```python
from build123d import *

# Parameters (mm, degrees)
F0_W      = 25.4
F0_H      = 25.580178
F2_DEPTH  = 25.4
F1_R      = 1.8161
F3_DEPTH  = 11.2776
F1_R_2    = 11.5316
F1_R_3    = 8.382
F4_DEPTH  = 3.7338
F1_R_4    = 4.9911
F5_DEPTH  = 8.8138
F6_DEPTH  = 6.1722
F7_R      = 1.8161
F12_DEPTH = 11.2776
F8_R      = 1.8161
F13_DEPTH = 11.2776
F9_R      = 1.8161
F14_DEPTH = 11.2776
F11_R     = 1.8161
F15_DEPTH = 11.2776
F10_R     = 1.8161
F16_DEPTH = 11.2776
F9_R_2    = 4.9911
F17_DEPTH = 8.8138
F11_R_2   = 4.9911
F18_DEPTH = 8.8138
F11_R_3   = 8.382
F19_DEPTH = 6.1722
F11_R_4   = 11.5316
F20_DEPTH = 3.7338
F21_DEPTH = 8.8138
F9_R_3    = 8.382
F22_DEPTH = 6.1722
F9_R_4    = 11.5316
F23_DEPTH = 3.7338
F10_R_2   = 4.9911
F24_DEPTH = 8.8138
F10_R_3   = 8.382
F25_DEPTH = 6.1722
F10_R_4   = 11.5316
F26_DEPTH = 3.7338
F8_R_2    = 4.9911
F27_DEPTH = 8.8138
F8_R_3    = 8.382
F28_DEPTH = 6.1722
F7_R_2    = 4.9911
F29_DEPTH = 8.8138
F7_R_3    = 8.382
F30_DEPTH = 6.1722
F7_R_4    = 11.5316
F31_DEPTH = 3.7338
F8_R_4    = 11.5316
F32_DEPTH = 3.7338


with BuildPart() as f2:
    # F0 (on Front) → F2 (new body)
    with BuildSketch(Plane.XZ):
        Rectangle(F0_W, F0_H)
    extrude(amount=-F2_DEPTH)

    # F1 (on Front) → F3 (cut)
    with BuildSketch(Plane.XZ):
        Circle(F1_R)
    extrude(amount=-F3_DEPTH, mode=Mode.SUBTRACT)

    # F1 (on Front) → F4 (cut)
    with BuildSketch(Plane.XZ):
        Circle(F1_R_2)
        Circle(F1_R_3, mode=Mode.SUBTRACT)
    extrude(amount=-F4_DEPTH, mode=Mode.SUBTRACT)

    # F1 (on Front) → F5 (cut)
    with BuildSketch(Plane.XZ):
        Circle(F1_R_4)
        Circle(F1_R, mode=Mode.SUBTRACT)
    extrude(amount=-F5_DEPTH, mode=Mode.SUBTRACT)

    # F1 (on Front) → F6 (cut)
    with BuildSketch(Plane.XZ):
        Circle(F1_R_3)
        Circle(F1_R_4, mode=Mode.SUBTRACT)
    extrude(amount=-F6_DEPTH, mode=Mode.SUBTRACT)

    # F7 (on face) → F12 (cut)
    with BuildSketch(Plane(origin=(-12.7, 0, 0), x_dir=(0, -1, 0), z_dir=(-1, 0, 0))):
        with Locations((-12.7, 0)):
            Circle(F7_R)
    extrude(amount=-F12_DEPTH, mode=Mode.SUBTRACT)

    # F8 (on face) → F13 (cut)
    with BuildSketch(Plane(origin=(0, 0, -12.790089), x_dir=(1, 0, 0), z_dir=(0, 0, -1))):
        with Locations((0, -12.7)):
            Circle(F8_R)
    extrude(amount=-F13_DEPTH, mode=Mode.SUBTRACT)

    # F9 (on face) → F14 (cut)
    with BuildSketch(Plane.XY.offset(12.790089)):
        with Locations((0, 12.7)):
            Circle(F9_R)
    extrude(amount=-F14_DEPTH, mode=Mode.SUBTRACT)

    # F11 (on face) → F15 (cut)
    with BuildSketch(Plane(origin=(0, 25.4, 0), x_dir=(-1, 0, 0), z_dir=(0, 1, 0))):
        Circle(F11_R)
    extrude(amount=-F15_DEPTH, mode=Mode.SUBTRACT)

    # F10 (on face) → F16 (cut)
    with BuildSketch(Plane.YZ.offset(12.7)):
        with Locations((12.7, 0)):
            Circle(F10_R)
    extrude(amount=-F16_DEPTH, mode=Mode.SUBTRACT)

    # F9 (on face) → F17 (cut)
    with BuildSketch(Plane.XY.offset(12.790089)):
        with Locations((0, 12.7)):
            Circle(F9_R_2)
        with Locations((0, 12.7)):
            Circle(F9_R, mode=Mode.SUBTRACT)
    extrude(amount=-F17_DEPTH, mode=Mode.SUBTRACT)

    # F11 (on face) → F18 (cut)
    with BuildSketch(Plane(origin=(0, 25.4, 0), x_dir=(-1, 0, 0), z_dir=(0, 1, 0))):
        Circle(F11_R_2)
        Circle(F11_R, mode=Mode.SUBTRACT)
    extrude(amount=-F18_DEPTH, mode=Mode.SUBTRACT)

    # F11 (on face) → F19 (cut)
    with BuildSketch(Plane(origin=(0, 25.4, 0), x_dir=(-1, 0, 0), z_dir=(0, 1, 0))):
        Circle(F11_R_3)
        Circle(F11_R_2, mode=Mode.SUBTRACT)
    extrude(amount=-F19_DEPTH, mode=Mode.SUBTRACT)

    # F11 (on face) → F20 (cut)
    with BuildSketch(Plane(origin=(0, 25.4, 0), x_dir=(-1, 0, 0), z_dir=(0, 1, 0))):
        Circle(F11_R_4)
        Circle(F11_R_3, mode=Mode.SUBTRACT)
    extrude(amount=-F20_DEPTH, mode=Mode.SUBTRACT)

    # F9 (on face) → F21 (cut)
    with BuildSketch(Plane.XY.offset(12.790089)):
        with Locations((0, 12.7)):
            Circle(F9_R_2)
        with Locations((0, 12.7)):
            Circle(F9_R, mode=Mode.SUBTRACT)
    extrude(amount=-F21_DEPTH, mode=Mode.SUBTRACT)

    # F9 (on face) → F22 (cut)
    with BuildSketch(Plane.XY.offset(12.790089)):
        with Locations((0, 12.7)):
            Circle(F9_R_3)
        with Locations((0, 12.7)):
            Circle(F9_R_2, mode=Mode.SUBTRACT)
    extrude(amount=-F22_DEPTH, mode=Mode.SUBTRACT)

    # F9 (on face) → F23 (cut)
    with BuildSketch(Plane.XY.offset(12.790089)):
        with Locations((0, 12.7)):
            Circle(F9_R_4)
        with Locations((0, 12.7)):
            Circle(F9_R_3, mode=Mode.SUBTRACT)
    extrude(amount=-F23_DEPTH, mode=Mode.SUBTRACT)

    # F10 (on face) → F24 (cut)
    with BuildSketch(Plane.YZ.offset(12.7)):
        with Locations((12.7, 0)):
            Circle(F10_R_2)
        with Locations((12.7, 0)):
            Circle(F10_R, mode=Mode.SUBTRACT)
    extrude(amount=-F24_DEPTH, mode=Mode.SUBTRACT)

    # F10 (on face) → F25 (cut)
    with BuildSketch(Plane.YZ.offset(12.7)):
        with Locations((12.7, 0)):
            Circle(F10_R_3)
        with Locations((12.7, 0)):
            Circle(F10_R_2, mode=Mode.SUBTRACT)
    extrude(amount=-F25_DEPTH, mode=Mode.SUBTRACT)

    # F10 (on face) → F26 (cut)
    with BuildSketch(Plane.YZ.offset(12.7)):
        with Locations((12.7, 0)):
            Circle(F10_R_4)
        with Locations((12.7, 0)):
            Circle(F10_R_3, mode=Mode.SUBTRACT)
    extrude(amount=-F26_DEPTH, mode=Mode.SUBTRACT)

    # F8 (on face) → F27 (cut)
    with BuildSketch(Plane(origin=(0, 0, -12.790089), x_dir=(1, 0, 0), z_dir=(0, 0, -1))):
        with Locations((0, -12.7)):
            Circle(F8_R_2)
        with Locations((0, -12.7)):
            Circle(F8_R, mode=Mode.SUBTRACT)
    extrude(amount=-F27_DEPTH, mode=Mode.SUBTRACT)

    # F8 (on face) → F28 (cut)
    with BuildSketch(Plane(origin=(0, 0, -12.790089), x_dir=(1, 0, 0), z_dir=(0, 0, -1))):
        with Locations((0, -12.7)):
            Circle(F8_R_3)
        with Locations((0, -12.7)):
            Circle(F8_R_2, mode=Mode.SUBTRACT)
    extrude(amount=-F28_DEPTH, mode=Mode.SUBTRACT)

    # F7 (on face) → F29 (cut)
    with BuildSketch(Plane(origin=(-12.7, 0, 0), x_dir=(0, -1, 0), z_dir=(-1, 0, 0))):
        with Locations((-12.7, 0)):
            Circle(F7_R_2)
        with Locations((-12.7, 0)):
            Circle(F7_R, mode=Mode.SUBTRACT)
    extrude(amount=-F29_DEPTH, mode=Mode.SUBTRACT)

    # F7 (on face) → F30 (cut)
    with BuildSketch(Plane(origin=(-12.7, 0, 0), x_dir=(0, -1, 0), z_dir=(-1, 0, 0))):
        with Locations((-12.7, 0)):
            Circle(F7_R_3)
        with Locations((-12.7, 0)):
            Circle(F7_R_2, mode=Mode.SUBTRACT)
    extrude(amount=-F30_DEPTH, mode=Mode.SUBTRACT)

    # F7 (on face) → F31 (cut)
    with BuildSketch(Plane(origin=(-12.7, 0, 0), x_dir=(0, -1, 0), z_dir=(-1, 0, 0))):
        with Locations((-12.7, 0)):
            Circle(F7_R_4)
        with Locations((-12.7, 0)):
            Circle(F7_R_3, mode=Mode.SUBTRACT)
    extrude(amount=-F31_DEPTH, mode=Mode.SUBTRACT)

    # F8 (on face) → F32 (cut)
    with BuildSketch(Plane(origin=(0, 0, -12.790089), x_dir=(1, 0, 0), z_dir=(0, 0, -1))):
        with Locations((0, -12.7)):
            Circle(F8_R_4)
        with Locations((0, -12.7)):
            Circle(F8_R_3, mode=Mode.SUBTRACT)
    extrude(amount=-F32_DEPTH, mode=Mode.SUBTRACT)


solid = f2.part
```
Can you work these out from the model? Positions are in its coordinate system, mm. A direction names the side the tool comes from. Coordinates: 2 decimals unless noted, no trailing zeros. Answer as a JSON object with one key per item and string values.
1) Thinking about a two-plate mould opening in Y: for faces 6 (the face through (0, 16.586, 2)), 7 (the face through (12.7, 13, -12)), 8 (the face through (3, 21, 9.056)), 9 (the face through (-4, 5, -9.056)), which applies, pulls with the +Y half, pulls with the -Y half, needs draft (parallel to the pull), parting line crosses it, or undercut?
Results:
{"face 6": "pulls with the +Y half", "face 7": "needs draft", "face 8": "undercut", "face 9": "undercut"}
2) For faces 1 (the face through (-3.96, 7.18, -3.04)), 2 (the face through (3.886, 13, 2)), 3 (the face through (3.96, 18.22, -3.04)), 4 (the face through (-2, 13, 3.976)), 5 (the face through (-8.374, 12.331, -8.667)), which set-ups out of +Z, -Z, +X, -X, +Y, -Y let a thin tool reach every point of the face, with its end or its side?
Results:
{"face 1": "-Y", "face 2": "+X", "face 3": "+Y", "face 4": "+Z", "face 5": "-Z"}
3) Imagine slicing it at A-A (x = 0). Count the separate pieces of the cut face and the enclosed holes in it, then the cut area to 3 significant figures.
Results:
{"separate pieces": "17", "enclosed holes": "0", "area": "43.9 mm^2"}
4) For P1, Ø8, axis at y = 11.5, z = -1.5, coming from the -X side; P2, Ø1, axis at x = 5.5, z = 3.5, coming from the +Y side; P3, Ø8, axis at y = 18, z = 4, coming from the -X side; P4, Ø8, axis at y = 4, z = 3, coming from the +X side, each with a flat end and sliding along its axis, tell me the tip position at first contact or that it passes through.
Results:
{"P1": "stops at x = -6.53", "P2": "stops at y = 19.23", "P3": "stops at x = -8.97", "P4": "stops at x = 12.7"}
5) If I drill on line 1 (Y direction, x = -5.95, z = 0); line 2 (Z direction, x = 2.1, y = 12.7); line 3 (X direction, y = 12.7, z = -5.25), over which ranges is the centre line in solid material (lowest first)?
Results:
{"line 1": "y = 6.17 to 7.71, 17.69 to 19.23", "line 2": "z = -3.98 to -1.82, 1.82 to 3.98", "line 3": "x = -6.53 to -4.99, 4.99 to 6.53"}
